Could you check a few things on this model? Use its own coordinates, in mm. A direction names the side the tool comes from. Round coordinates to 2 decimals unless told otherwise and drop trailing zeros. Loops run counter-clockwise (first coordinate to the right, second up) from the corner with the lowest first, then second, coordinate; pieces in that order, holes last.
from build123d import *

# Parameters (mm, degrees)
F2_R     = 2.75
F3_DEPTH = 10


with BuildPart() as f1:
    # F0 (on Right) → F1 (revolve)
    with BuildSketch(Plane.YZ):
        Polygon((-7.162217, 3), (8.837783, 3), (8.837783, 7.5), (6.837783, 7.5), (6.837783, 25), (8.837783, 25), (8.837783, 44.3844), (-1.162217, 44.3844), (-1.162217, 27.719139), (-2.162217, 28.296489), (-7.162217, 28.296489), align=None)
    revolve(axis=Axis((0, 14.665759, 0), (0, 1, 0)))

    # F2 (on face) → F3 (cut, through all)
    with BuildSketch(Plane(origin=(0, 8.837783, 0), x_dir=(-1, 0, 0), z_dir=(0, 1, 0))):
        with BuildLine():
            ThreePointArc((-33.402795, 10.45243), (-28.494043, 20.324603), (-20.757853, 28.179985))
            ThreePointArc((-20.757853, 28.179985), (-19.797183, 29.663761), (-20.057996, 31.412033))
            ThreePointArc((-20.057996, 31.412033), (-20.54103, 37.056805), (-16.626689, 41.152499))
            ThreePointArc((-16.626689, 41.152499), (-36.134029, 25.774152), (-44.323573, 2.3229))
            ThreePointArc((-44.323573, 2.3229), (-41.725403, 7.35741), (-36.230905, 8.73845))
            ThreePointArc((-36.230905, 8.73845), (-34.492969, 9.061028), (-33.402795, 10.45243))
        make_face()
        with BuildLine():
            ThreePointArc((-36.945845, -4.903419), (-42.265885, -2.955613), (-44.323573, 2.3229))
            ThreePointArc((-44.323573, 2.3229), (-39.189099, -20.837214), (-22.859656, -38.044856))
            ThreePointArc((-22.859656, -38.044856), (-26.085097, -33.387249), (-24.724973, -27.887537))
            ThreePointArc((-24.724973, -27.887537), (-24.193881, -26.201589), (-24.91061, -24.585799))
            ThreePointArc((-24.91061, -24.585799), (-30.903166, -16.431505), (-34.312387, -6.903627))
            ThreePointArc((-34.312387, -6.903627), (-35.251149, -5.405894), (-36.945845, -4.903419))
        make_face()
        with BuildLine():
            ThreePointArc((-13.015562, -34.923261), (-17.23298, -38.706138), (-22.859656, -38.044856))
            ThreePointArc((-22.859656, -38.044856), (0, -44.3844), (22.859656, -38.044856))
            ThreePointArc((22.859656, -38.044856), (17.23298, -38.706138), (13.015562, -34.923261))
            ThreePointArc((13.015562, -34.923261), (11.776291, -33.66283), (10.013149, -33.537097))
            ThreePointArc((10.013149, -33.537097), (0, -35), (-10.013149, -33.537097))
            ThreePointArc((-10.013149, -33.537097), (-11.776291, -33.66283), (-13.015562, -34.923261))
        make_face()
        with BuildLine():
            ThreePointArc((44.3844, 0), (44.369191, 1.161848), (44.323573, 2.3229))
            ThreePointArc((44.323573, 2.3229), (42.265885, -2.955613), (36.945845, -4.903419))
            ThreePointArc((36.945845, -4.903419), (35.251149, -5.405894), (34.312387, -6.903627))
            ThreePointArc((34.312387, -6.903627), (30.903166, -16.431505), (24.91061, -24.585799))
            ThreePointArc((24.91061, -24.585799), (24.193881, -26.201589), (24.724973, -27.887537))
            ThreePointArc((24.724973, -27.887537), (26.085097, -33.387249), (22.859656, -38.044856))
            ThreePointArc((22.859656, -38.044856), (38.630215, -21.855924), (44.3844, 0))
        make_face()
        with BuildLine():
            ThreePointArc((44.323573, 2.3229), (36.134029, 25.774152), (16.626689, 41.152499))
            ThreePointArc((16.626689, 41.152499), (20.54103, 37.056805), (20.057996, 31.412033))
            ThreePointArc((20.057996, 31.412033), (19.797183, 29.663761), (20.757853, 28.179985))
            ThreePointArc((20.757853, 28.179985), (28.494043, 20.324603), (33.402795, 10.45243))
            ThreePointArc((33.402795, 10.45243), (34.492969, 9.061028), (36.230905, 8.73845))
            ThreePointArc((36.230905, 8.73845), (41.725403, 7.35741), (44.323573, 2.3229))
        make_face()
        with BuildLine():
            ThreePointArc((16.626689, 41.152499), (0, 44.3844), (-16.626689, 41.152499))
            ThreePointArc((-16.626689, 41.152499), (-10.965839, 40.925433), (-7.392117, 36.52938))
            ThreePointArc((-7.392117, 36.52938), (-6.365278, 35.090603), (-4.643513, 34.690601))
            ThreePointArc((-4.643513, 34.690601), (0, 35), (4.643513, 34.690601))
            ThreePointArc((4.643513, 34.690601), (6.365278, 35.090603), (7.392117, 36.52938))
            ThreePointArc((7.392117, 36.52938), (10.965839, 40.925433), (16.626689, 41.152499))
        make_face()
        with Locations((-14.047747, 34.769395)):
            Circle(F2_R)
        with Locations((14.047747, 34.769395)):
            Circle(F2_R)
        with Locations((37.448608, 1.962598)):
            Circle(F2_R)
        with Locations((19.313928, -32.143774)):
            Circle(F2_R)
        with Locations((-19.313928, -32.143774)):
            Circle(F2_R)
        with Locations((-37.448608, 1.962598)):
            Circle(F2_R)
    extrude(amount=-F3_DEPTH, mode=Mode.SUBTRACT)


solid = f1.part
Item 1: If we section it at D-D, the plane y = 3.75: Count the separate pieces of the cut face and the enclosed holes in it, then the cut area to 3 significant figures.
Results list:
separate pieces: 1
enclosed holes: 7
area: 4,360 mm2
Item 2: For faces 1 (the cylindrical face through (0, 4, 35)), 2 (the cylindrical face through (0.33, 7.824, -7.493)), which set-ups out of +Z, -Z, +X, -X, +Y, -Y let a thin tool reach every point of the face, with its end or its side?
Results list:
face 1: +Z, +Y, -Y
face 2: +Y
Item 3: If we section it at C-C, the plane x = 38: Please give me the cut outline in (y, z).
Results list:
outline: (-1.16, -4.9) - (8.84, -4.9) - (8.84, -0.73) - (-1.16, -0.73) - close; (-1.16, 4.66) - (8.84, 4.66) - (8.84, 8.82) - (-1.16, 8.82) - close
Item 4: If we section it at B-B, the plane y = -5: Please give me the cut outline in (x, z).
Results list:
outline: circle Ø56.59 at (0, 0); hole circle Ø6 at (0, 0)
Item 5: Will these pins go through, and if not, where does the flat tip stop? pin 1 (3 mm diameter, centred on y = -3.5, z = 19.5, fed in from -X); pin 2 (1 mm diameter, centred on x = -15.5, y = -4.5, fed in from +Z); pin 3 (7 mm diameter, centred on x = -19.31, z = -32.14, fed in from -Y); pin 4 (3 mm diameter, centred on x = 34.5, z = -11, fed in from +Y).
Results list:
pin 1: stops at x = -21.83
pin 2: stops at z = 23.99
pin 3: stops at y = -1.16
pin 4: stops at y = 8.84
Item 6: If I drill on line 1 along X through (y, z) = (4.75, 0); line 2 along X through (y, z) = (7.8, 0); line 3 along X through (y, z) = (4, 36), over which ranges is the centre line in solid material (lowest first)?
Results list:
line 1: x = -44.05 to -39.37, -35.52 to -3, 3 to 35.52, 39.37 to 44.05
line 2: x = -44.05 to -39.37, -35.52 to -25, -7.5 to -3, 3 to 7.5, 25 to 35.52, 39.37 to 44.05
line 3: x = -20.82 to -16.51, -11.59 to -7.19, 7.19 to 11.59, 16.51 to 20.82
Item 7: We'd pull the mould along Z, two halves only. Please class faces 3 (the cylindrical face through (34.51, 3.91, 9.05)), 4 (the cylindrical face through (0, 4, -35)), 5 (the cylindrical face through (-19.79, 3.91, 29.69)): released by +Z, released by -Z, zero draft, split by the parting line, or undercut.
Results list:
face 3: released by +Z
face 4: released by -Z
face 5: undercut
Item 8: If we section it at A-A, the plane x = 0: Please give me the cut outline in (y, z), then the cut area to 3 significant figures.
Results list:
outline: (-7.16, -28.3) - (-2.16, -28.3) - (-1.16, -27.72) - (-1.16, -35) - (8.84, -35) - (8.84, -25) - (6.84, -25) - (6.84, -7.5) - (8.84, -7.5) - (8.84, -3) - (-7.16, -3) - close; (-7.16, 3) - (8.84, 3) - (8.84, 7.5) - (6.84, 7.5) - (6.84, 25) - (8.84, 25) - (8.84, 35) - (-1.16, 35) - (-1.16, 27.72) - (-2.16, 28.3) - (-7.16, 28.3) - close
area: 873 mm2
